Build history of the part. All positions in model axes, mm. A direction names the side the tool comes from. Round coordinates to 2 decimals unless told otherwise and drop trailing zeros. Order: outer loops, then holes, each group sorted by start corner. A loop starts at its lowest first (then second) coordinate and runs counter-clockwise, first axis right, second up. Notation, with made-up numbers: (46, -39) -> (91, -39) arc R31 cw to (91, 0) -> close; hole circle Ø3 at (84, 37). An arc over 180 degrees is marked (long way). Write item = value, one per line.
from build123d import *

# Parameters (mm, degrees)
F1_DEPTH = 15
F3_D     = 60
F4_D     = 30
F6_DEPTH = 5
F8_DEPTH = 5


with BuildPart() as f1:
    # F0 (on Top) → F1 (new body)
    with BuildSketch(Plane.XY):
        with BuildLine():
            Line((203, 29.8496231132), (5, 49.7493718553))
            ThreePointArc((5, 49.7493718553), (-50, 0), (5, -49.7493718553))
            Line((5, -49.7493718553), (203, -29.8496231132))
            ThreePointArc((203, -29.8496231132), (230, 0), (203, 29.8496231132))
        make_face()
    extrude(amount=F1_DEPTH)

    # F3 (through all)
    with Locations(Plane(origin=(0, 0, 0), x_dir=(1, 0, 0), z_dir=(0, 0, -1))):
        with Locations((0, 0)):
            Hole(F3_D / 2)

    # F4 (through all)
    with Locations(Plane(origin=(0, 0, 0), x_dir=(1, 0, 0), z_dir=(0, 0, -1))):
        with Locations((200, 0)):
            Hole(F4_D / 2)

    # F5 (on face) → F6 (cut)
    with BuildSketch(Plane.XY.offset(15)):
        with BuildLine():
            Line((168.6271068081, 23.2538507084), (43.7994974843, 35.7994974843))
            ThreePointArc((43.7994974843, 35.7994974843), (34.3472728952, 31.1937693965), (34.2395979874, 20.6796984906))
            ThreePointArc((34.2395979874, 20.6796984906), (40, 0), (34.2395979874, -20.6796984906))
            ThreePointArc((34.2395979874, -20.6796984906), (34.3472728952, -31.1937693965), (43.7994974843, -35.7994974843))
            Line((43.7994974843, -35.7994974843), (168.6271068081, -23.2538507084))
            ThreePointArc((168.6271068081, -23.2538507084), (176.2023684566, -18.4483798654), (176.8765048629, -9.5028402409))
            ThreePointArc((176.8765048629, -9.5028402409), (175, 0), (176.8765048629, 9.5028402409))
            ThreePointArc((176.8765048629, 9.5028402409), (176.2023684566, 18.4483798654), (168.6271068081, 23.2538507084))
        make_face()
    extrude(amount=-F6_DEPTH, mode=Mode.SUBTRACT)

    # F7 (on Top) → F8 (cut)
    with BuildSketch(Plane.XY):
        with BuildLine():
            Line((168.6271068081, 23.2538507084), (43.7994974843, 35.7994974843))
            ThreePointArc((43.7994974843, 35.7994974843), (34.3472728952, 31.1937693965), (34.2395979874, 20.6796984906))
            ThreePointArc((34.2395979874, 20.6796984906), (40, 0), (34.2395979874, -20.6796984906))
            ThreePointArc((34.2395979874, -20.6796984906), (34.3472728952, -31.1937693965), (43.7994974843, -35.7994974843))
            Line((43.7994974843, -35.7994974843), (168.6271068081, -23.2538507084))
            ThreePointArc((168.6271068081, -23.2538507084), (176.2023684566, -18.4483798654), (176.8765048629, -9.5028402409))
            ThreePointArc((176.8765048629, -9.5028402409), (175, 0), (176.8765048629, 9.5028402409))
            ThreePointArc((176.8765048629, 9.5028402409), (176.2023684566, 18.4483798654), (168.6271068081, 23.2538507084))
        make_face()
    extrude(amount=F8_DEPTH, mode=Mode.SUBTRACT)


solid = f1.part
Q1. Mould opens along X. For faces 1 (the face through (34.43, 31.32, 12.54)), 2 (the face through (88, -33, 15)), 3 (the face through (102.61, -39.94, 7.4)) say: released by +X, released by -X, zero draft, split by the parting line, or undercut.
Check values:
face_1 = undercut
face_2 = zero draft
face_3 = released by +X
Q2. Flat gauge pins, fed straight in: pin 1 (8 mm diameter, centred on x = 48, z = 8, fed in from +Y); pin 2 (24 mm diameter, centred on x = 200, y = 0, fed in from +Z); pin 3 (6 mm diameter, centred on x = 41, y = 20.5, fed in from +Z); pin 4 (1.5 mm diameter, centred on x = 165, z = 7, fed in from -Y). Where does each tip first touch, or does it go through?
Check values:
pin_1 = 45.83
pin_2 = through
pin_3 = 10
pin_4 = -33.74
Q3. Cut at D-D, the plane x = 200. List the corners of the cut face in (y, z).
Check values:
outline = (-30.15, 0) -> (-15, 0) -> (-15, 15) -> (-30.15, 15) -> close; (15, 0) -> (30.15, 0) -> (30.15, 15) -> (15, 15) -> close
Q4. Cut at A-A, the plane y = 0. List the corners of the cut face in (x, z).
Check values:
outline = (-50, 0) -> (-30, 0) -> (-30, 15) -> (-50, 15) -> close; (30, 0) -> (40, 0) -> (40, 5) -> (175, 5) -> (175, 0) -> (185, 0) -> (185, 15) -> (175, 15) -> (175, 10) -> (40, 10) -> (40, 15) -> (30, 15) -> close; (215, 0) -> (230, 0) -> (230, 15) -> (215, 15) -> close
Q5. Probe probe 1 along Y at (x, z) = (0, 3); probe 2 along Y at (x, z) = (37, 2.25); probe 3 along X at (y, z) = (-21, 12.5). List the from-to ranges inside material, lowest first.
Check values:
probe_1 = -50 to -30, 30 to 50
probe_2 = -46.53 to -34, -15.2 to 15.2, 34 to 46.53
probe_3 = -45.38 to -21.42, 21.42 to 34.05, 174.01 to 221.42
Q6. Which spindle directions (+Z, -Z, +X, -X, +Y, -Y) get a long thin tool onto all of the face, cutting with end or side? Do faces 4 (the face through (105.39, 39.66, 7.4)), 5 (the face through (175, 0, 2)), 6 (the face through (34.265, -31.062, 12.535)). Say none if no direction does.
Check values:
face_4 = +Z, -Z, +X, +Y
face_5 = -Z
face_6 = +Z
Q7. Cut at B-B, the plane x = 0. List the corners of the cut face in (y, z), and give its area (3 significant figures).
Check values:
outline = (-50, 0) -> (-30, 0) -> (-30, 15) -> (-50, 15) -> close; (30, 0) -> (50, 0) -> (50, 15) -> (30, 15) -> close
area = 600 mm²
Q8. Cut at C-C, the plane x = 121. List the corners of the cut face in (y, z), and give its area (3 significant figures).
Check values:
outline = (-38.09, 0) -> (-28.04, 0) -> (-28.04, 5) -> (28.04, 5) -> (28.04, 0) -> (38.09, 0) -> (38.09, 15) -> (28.04, 15) -> (28.04, 10) -> (-28.04, 10) -> (-28.04, 15) -> (-38.09, 15) -> close
area = 582 mm²
